Read the model definition and answer for the solid it produces. Units are mm, in the model's axes. Face numbers are marked on the shaded views. A direction names the side the tool comes from. Coordinates: 2 decimals unless noted, no trailing zeros. Loops run counter-clockwise (first coordinate to the right, second up) from the corner with the lowest first, then second, coordinate; pieces in that order, holes last. Notation, with made-up numbers: (44.5, 41) - (93.5, 41) arc R34 cw to (93.5, 73) - close; hole circle Ø6 at (84, 16). An arc over 180 degrees is marked (long way). Use one line per item in the form item = value. Start each with the question number.
1) Which of the six approach directions +Z, -Z, +X, -X, +Y, -Y give full straight-line access (tool end or side, diameter ignored) to the marked faces 4 and 5?
2) A cutting plane is placed at A-A (x = 5). Give the vertices of the cut face in (y, z), and give its area (3 significant figures).
3) The mould has two halves that part along X. Classify the marked faces 1, 2 and 3: released by +X, released by -X, zero draft, split by the parting line, or undercut.
4) A cutting plane is placed at C-C (z = 10). Give the vertices of the cut face in (x, y) (1 decimal), and give its area (3 significant figures).
5) Consider line 1 (Y direction, x = -35, z = 73); line 2 (X direction, y = -42, z = -121.5). Determine where each line is inside the solid, lowest interval first.
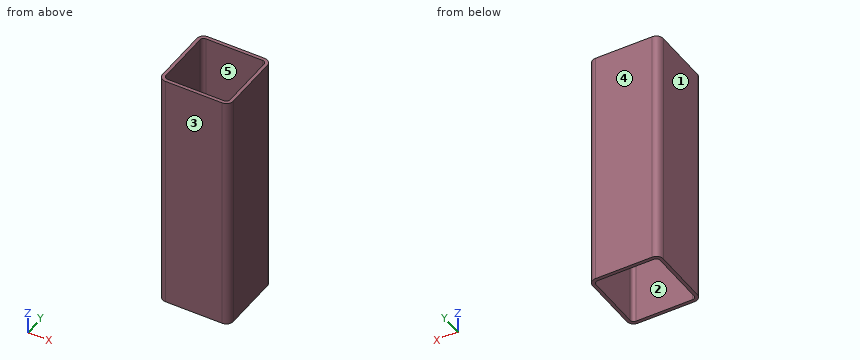
from build123d import *

# Parameters (mm, degrees)
F1_DEPTH = 175


with BuildPart() as f1:
    # F0 (on Top) → F1 (new body, symmetric)
    with BuildSketch(Plane.XY):
        with BuildLine():
            Line((40.8, 50.8), (-40.8, 50.8))
            ThreePointArc((-40.8, 50.8), (-47.871068, 47.871068), (-50.8, 40.8))
            Line((-50.8, 40.8), (-50.8, -40.8))
            ThreePointArc((-50.8, -40.8), (-47.871068, -47.871068), (-40.8, -50.8))
            Line((-40.8, -50.8), (40.8, -50.8))
            ThreePointArc((40.8, -50.8), (47.871068, -47.871068), (50.8, -40.8))
            Line((50.8, -40.8), (50.8, 40.8))
            ThreePointArc((50.8, 40.8), (47.871068, 47.871068), (40.8, 50.8))
        make_face()
        with BuildLine():
            ThreePointArc((-46.0375, 40.8), (-44.503472, 44.503472), (-40.8, 46.0375))
            Line((-40.8, 46.0375), (40.8, 46.0375))
            ThreePointArc((40.8, 46.0375), (44.503472, 44.503472), (46.0375, 40.8))
            Line((46.0375, 40.8), (46.0375, -40.8))
            ThreePointArc((46.0375, -40.8), (44.503472, -44.503472), (40.8, -46.0375))
            Line((40.8, -46.0375), (-40.8, -46.0375))
            ThreePointArc((-40.8, -46.0375), (-44.503472, -44.503472), (-46.0375, -40.8))
            Line((-46.0375, -40.8), (-46.0375, 40.8))
        make_face(mode=Mode.SUBTRACT)
    extrude(amount=F1_DEPTH, both=True)


solid = f1.part
Found:
q1.face_4 = +Z, -Z, +X, -X, +Y
q1.face_5 = +Z, -Z
q2.outline = (-50.8, -175) - (-46.04, -175) - (-46.04, 175) - (-50.8, 175) - close; (46.04, -175) - (50.8, -175) - (50.8, 175) - (46.04, 175) - close
q2.area = 3,330 mm^2
q3.face_1 = released by -X
q3.face_2 = undercut
q3.face_3 = zero draft
q4.outline = (-50.8, -40.8) arc R10 ccw to (-40.8, -50.8) - (40.8, -50.8) arc R10 ccw to (50.8, -40.8) - (50.8, 40.8) arc R10 ccw to (40.8, 50.8) - (-40.8, 50.8) arc R10 ccw to (-50.8, 40.8) - close; hole (-46, -40.8) arc R5.2 ccw to (-40.8, -46) - (40.8, -46) arc R5.2 ccw to (46, -40.8) - (46, 40.8) arc R5.2 ccw to (40.8, 46) - (-40.8, 46) arc R5.2 ccw to (-46, 40.8) - close
q4.area = 1,780 mm^2
q5.line_1 = -50.8 to -46.04, 46.04 to 50.8
q5.line_2 = -50.73 to -45.9, 45.9 to 50.73
